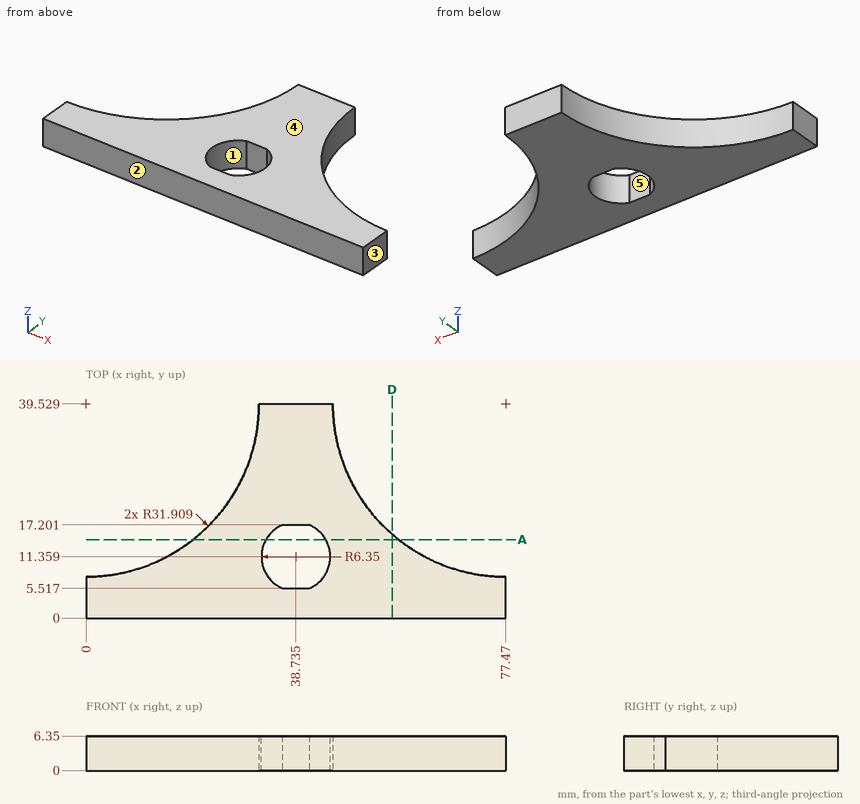
Drawing for the job (mm, zero at the part's lowest x, y, z). A direction names the side the tool comes from. Give positions to 0.01 mm unless a question says otherwise; leave off trailing zeros. Loops run counter-clockwise (first coordinate to the right, second up) from the corner with the lowest first, then second, coordinate; pieces in that order, holes last. Notation, with made-up numbers: M 9,63.25 L 28,63.25 A18 ccw 28,90.25 Z; hole C 13.5,10 d4. An arc over 180 degrees is marked long. Use one line per item in the form item = value.
Item 1: Which spindle directions (+Z, -Z, +X, -X, +Y, -Y) get a long thin tool onto all of the face, cutting with end or side? Do the marked faces 1 and 2. Say none if no direction does.
Determined:
face_1 = +Z, -Z
face_2 = +Z, -Z, +X, -X, -Y
Item 2: Slice it at D-D (x = 56.5). List the corners of the cut face in (y, z), plus the area to 3 significant figures.
Determined:
outline = M 0,0 L 15.48,0 L 15.48,6.35 L 0,6.35 Z
area = 98.3 mm2
Item 3: Two-plate mould, pull along X, no slides. Class the marked faces 3, 4 and 5: pulls with the +X half, pulls with the -X half, needs draft (parallel to the pull), parting line crosses it, or undercut.
Determined:
face_3 = pulls with the +X half
face_4 = needs draft
face_5 = undercut
Item 4: Flat gauge pins, fed straight in: pin 1 (3 mm diameter, centred on x = 46.5, z = 0.5, fed in from -Y); pin 2 (2 mm diameter, centred on x = 65, z = 4, fed in from +Y); pin 3 (8 mm diameter, centred on x = 23, y = 24.5, fed in from -Z); pin 4 (1 mm diameter, centred on y = 22.5, z = 3.5, fed in from -X). Where does each tip first touch, or does it go through?
Determined:
pin_1 = 0
pin_2 = 10.6
pin_3 = through
pin_4 = 26.66
Item 5: Slice it at A-A (y = 14.5). List the corners of the cut face in (x, z).
Determined:
outline = M 19.79,0 L 33.22,0 L 33.22,6.35 L 19.79,6.35 Z; M 44.25,0 L 57.68,0 L 57.68,6.35 L 44.25,6.35 Z
Item 6: Drill centre lines: probe 1 along X at (y, z) = (14.5, 5.5) (1 decimal); probe 2 along X at (y, z) = (11, 3.75) (1 decimal); probe 3 along X at (y, z) = (27, 4.5). Where is each one in solid material? Low to high. Write a range as from..to.
Determined:
probe_1 = 19.8..33.2, 44.3..57.7
probe_2 = 14.3..32.4, 45.1..63.2
probe_3 = 29.35..48.12
